The listing builds one solid part. Answer for the finished solid, in the listing's coordinates (mm). Face numbers are marked on the shaded views. Coordinates: 2 decimals unless noted, no trailing zeros. Loops run counter-clockwise (first coordinate to the right, second up) from the corner with the lowest first, then second, coordinate; pieces in that order, holes last. Notation, with made-up numbers: M 47.25,-0.75 L 94.25,-0.75 A13 cw 94.25,13.25 Z; hole C 47.5,58.5 d10. An arc over 180 degrees is marked long. Return JSON: item names as keys, results as strings. Group by question number.
1. Straight lines are drawn through the part: L1, parallel to Z at x = 25, y = 0; L2, parallel to Y at x = 0, z = 22.65; L3, parallel to Y at x = 25.15, z = 49. For each, find the intervals that lie inside material, in ascending order. Write a range as from..to.
2. Section B-B (z = 20) is taken. Write down the section's boundary in (x, y), then the cut area to 3 significant figures.
3. Given P1, Ø1.5, axis at x = 19, y = 6.5, coming from the +Z side; P2, Ø10, axis at y = -17.5, z = 17.5, coming from the +X side; P3, Ø6, axis at y = 0.5, z = 43, coming from the +X side, each flat-ended and moving along its own axis, determine where each tip first touches the part or whether it passes through.
4. Section C-C (x = 33) is taken. Write down the section's boundary in (y, z).
5. The mould has two halves that part along X. Classify the marked faces 1 and 2: pulls with the +X half, pulls with the -X half, needs draft (parallel to the pull), parting line crosses it, or undercut.
6. Section A-A (y = 0) is taken. Count the separate pieces of the cut face and the enclosed holes in it, then the cut area to 3 significant figures.
Autodesk Inventor part; units mm, degrees
ref_plane "YZ Plane" through (0, 0, 0) normal (1, 0, 0) x (0, 1, 0)
ref_plane "XZ Plane" through (0, 0, 0) normal (0, 1, 0) x (-1, 0, 0)
ref_plane "XY Plane" through (0, 0, 0) normal (0, 0, 1) x (1, 0, 0)
sketch "Sketch1" plane through (0, 0, 0) normal (0, 1, 0) x (-1, 0, 0)
  line L0 (0, 0) -> (0, 24.5)
  line L1 (26.6502, 0) -> (0, 0)
  line L2 (0, 24.5) -> (26.3718, 24.5)
  line L3 (23.9, 22) -> (24.15, 0)
  line L4 (26.6502, 0) -> (26.3718, 24.5)
  line L5 (20, 24.5) -> (20, 22)
  line L6 (20, 22) -> (23.9, 22)
  line L7 (20, 22) -> (0, 22) construction
  dimension "d0" = 48.3
  dimension "d3" = 47.8
  dimension "d4" = 2.5
  dimension "d5" = 22
  dimension "d6" = 2.5
  dimension "d7" = 40
revolve "Revolution1" add sketch "Sketch1" angle 360 about axis through (0, 0, 0) along (0, 0, 1) contours L3 L6 L5 L2 L4 L1
sketch "Sketch2" plane through (0, 0, 24.5) normal (0, 0, 1) x (1, 0, 0)
  circle A0 centre (0, 0) radius 26.3718
  circle A1 centre (0, 0) radius 20
  circle A2 centre (0, 0) radius 22.7
  circle A3 centre (0, 0) radius 20
  dimension "d8" = 40
  dimension "d9" = 2.7
sketch "Sketch3" plane through (0, 0, 0) normal (0, 1, 0) x (-1, 0, 0)
  arc A0 (0, 24.5) -> (-24.5, 49) centre (-24.5, 24.5) ccw
  dimension "d10" = 24.5
  dimension "d11" = 24.5
  dimension "d12" = 24.5
sweep "Sweep1" add profiles "Sketch2" path "Sketch3" contours A2
sketch "Sketch4" plane through (0, 0, 0) normal (0, 1, 0) x (-1, 0, 0)
  line L0 (-24.5, 29) -> (-24.5, 69)
  line L1 (-49, 49) -> (-24.5, 49)
  line L2 (-24.5, 49) -> (-24.5, 75.5718)
  line L3 (-24.5, 75.5718) -> (-49, 75.8502)
  line L4 (-49, 75.8502) -> (-49, 49)
  line L5 (-49, 73.15) -> (-27, 72.9)
  line L6 (-27, 75.6002) -> (-27, 69)
  line L7 (-27, 69) -> (-24.5, 69)
  line L8 (-27, 69) -> (-27, 49) construction
  dimension "d14" = 2.7
  dimension "d15" = 22
  dimension "d16" = 2.5
  dimension "d17" = 48.3
  dimension "d18" = 47.8
  dimension "d19" = 40
revolve "Revolution2" add sketch "Sketch4" angle 360 about axis through (49, 0, 49) along (-1, 0, 0) contours L7 L6 L3 L2 | L4 L3 L6 L5
equation "\"d0\" = d1"
equation "\"d3\" = d2"
equation "\"d4\" = t2"
equation "\"d5\" = l1"
equation "\"d6\" = t2"
equation "\"d7\" = d"
equation "\"d8\" = d"
equation "\"d9\" = t1"
equation "\"d10\" = Z - t2"
equation "\"d11\" = Z - t2"
equation "\"d12\" = Z - t2"
equation "\"d14\" = t1"
equation "\"d15\" = l1"
equation "\"d16\" = t2"
equation "\"d17\" = d1"
equation "\"d18\" = d2"
equation "\"d19\" = d"
equation "\"d\" = 40"
equation "\"d1\" = 48.3"
equation "\"d2\" = 47.8"
equation "\"l1\" = 22"
equation "\"L\" = 49"
equation "\"t1\" = 2.7"
equation "\"t2\" = 2.5"
equation "\"Z\" = 27"
properties part number "JIS K 6739 90 Deg Elbow (DL) 40" material "PVC, Unplasticized"
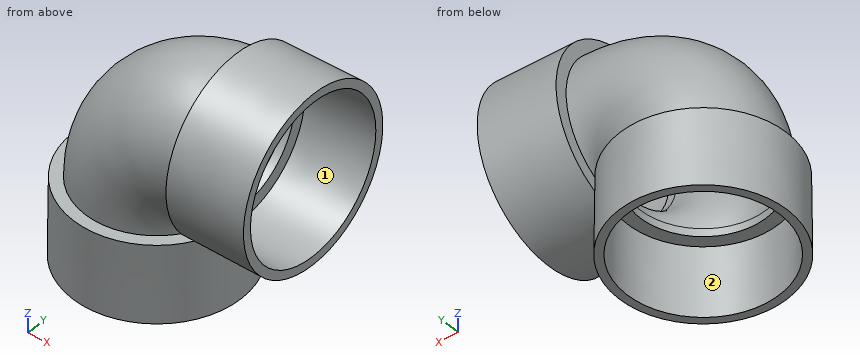
Worked out:
{
 "1": {"L1": "0..29, 69..75.58", "L2": "-26.39..-20, 20..26.39", "L3": "-26.58..-20, 20..26.58"},
 "2": {"outline": "C 0,0 d52.85; hole C 0,0 d47.85", "area": "395 mm^2"},
 "3": {"P1": "z = 70.65", "P2": "x = 23.31", "P3": "x = -14.45"},
 "4": {"outline": "C 0,49 d53.34; hole C 0,49 d47.94"},
 "5": {"face 1": "pulls with the +X half", "face 2": "undercut"},
 "6": {"separate pieces": "2", "enclosed holes": "1", "area": "498 mm^2"}
}
